```python
from build123d import *

# Parameters (mm, degrees)
SKETCH1_R           = 5
BOSS_EXTRUDE1_DEPTH = 20
SKETCH2_R           = 10
BOSS_EXTRUDE2_DEPTH = 2
SKETCH3_OUTSIDE_W   = 29.166
SKETCH3_OUTSIDE_H   = 29.166
CUT_EXTRUDE1_DEPTH  = 2


with BuildPart() as part:
    # Sketch1 → Boss-Extrude1 (new body)
    with BuildSketch(Plane(origin=(0, 0, 0), x_dir=(1, 0, 0), z_dir=(0, 1, 0))):
        Circle(SKETCH1_R)
    extrude(amount=BOSS_EXTRUDE1_DEPTH)

    # Sketch2 → Boss-Extrude2 (add)
    with BuildSketch(Plane(origin=(0, 20, 0), x_dir=(1, 0, 0), z_dir=(0, 1, 0))):
        Circle(SKETCH2_R)
    extrude(amount=BOSS_EXTRUDE2_DEPTH)

    # Sketch3 outside → Cut-Extrude1 (cut)
    with BuildSketch(Plane(origin=(0, 22, 0), x_dir=(1, 0, 0), z_dir=(0, 1, 0))):
        Rectangle(SKETCH3_OUTSIDE_W, SKETCH3_OUTSIDE_H)
        Polygon((0, 10), (8.660254038, 5), (8.660254038, -5), (0, -10), (-8.660254038, -5), (-8.660254038, 5), align=None, mode=Mode.SUBTRACT)
    extrude(amount=-CUT_EXTRUDE1_DEPTH, mode=Mode.SUBTRACT)


solid = part.part
```
Check sheet for the modelled part. Datum: model origin and axes. Units: mm. A direction names the side the tool comes from. Coordinates: 2 decimals unless noted, no trailing zeros. Loops run counter-clockwise (first coordinate to the right, second up) from the corner with the lowest first, then second, coordinate; pieces in that order, holes last.
1) Sectioned sample at B-B (x = 0.5). Record the boundary of the cut face in (y, z), and give its area (3 significant figures).
2) Sectioned sample at A-A (z = 0). Record the boundary of the cut face in (x, y), and give its area (3 significant figures).
3) Gauge pin test, flat ends, axial feed: pin 1 (5 mm diameter, centred on x = 1.5, y = 15, fed in from -Z); pin 2 (1 mm diameter, centred on x = -3.5, y = 17, fed in from +Z); pin 3 (1 mm diameter, centred on y = 15, z = -4.5, fed in from -X). Record the tip position at first contact, or that the pin passes through.
4) Sectioned sample at C-C (y = 6.75). Record the boundary of the cut face in (x, z).
5) Material ranges on probe 1 along Y at (x, z) = (-6, 1.75); probe 2 along Z at (x, y) = (1.5, 14), recorded low to high.
6) Sectioned sample at D-D (z = 8.75). Record the boundary of the cut face in (x, y), and give its area (3 significant figures).
7) Access from +Z, -Z, +X, -X, +Y, -Y to the whole of each face (thin tool, end or side, straight path). Record for faces 1 (the face through (-1.08, 9.86, 4.88)), 2 (the face through (-4.391, 21.014, -7.465)).
Check sheet entries:
1. outline: (0, -4.97) - (20, -4.97) - (20, -9.71) - (22, -9.71) - (22, 9.71) - (20, 9.71) - (20, 4.97) - (0, 4.97) - close
1. area: 238 mm2
2. outline: (-8.66, 20) - (-5, 20) - (-5, 0) - (5, 0) - (5, 20) - (8.66, 20) - (8.66, 22) - (-8.66, 22) - close
2. area: 235 mm2
3. pin 1: stops at z = -5
3. pin 2: stops at z = 4
3. pin 3: stops at x = -3
4. outline: circle Ø10 at (0, 0)
5. probe 1: y = 20 to 22
5. probe 2: z = -4.77 to 4.77
6. outline: (-2.17, 20) - (2.17, 20) - (2.17, 22) - (-2.17, 22) - close
6. area: 8.66 mm2
7. face 1: -Y
7. face 2: -Z, -X, +Y, -Y
